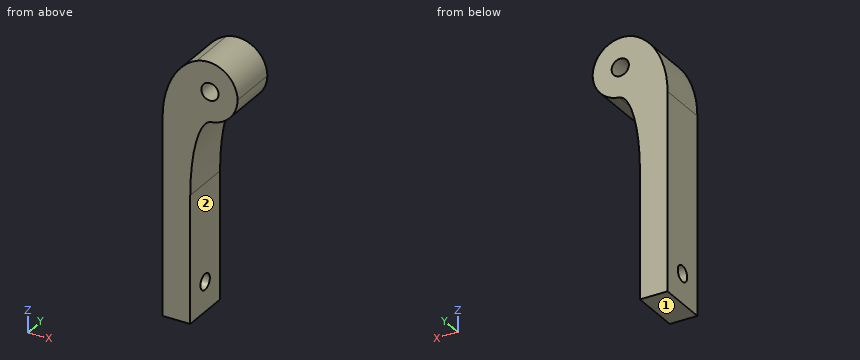
from build123d import *

# Parameters (mm, degrees)
SKETCH1_W               = 7
SKETCH1_H               = 52
BOSS_EXTRUDE1_DEPTH     = 12.7
SKETCH2_R               = 2
CUT_EXTRUDE1_DEPTH      = 10
SKETCH3_W               = 24
SKETCH3_H               = 15
BOSS_EXTRUDE2_DEPTH     = 12.7
CUT_EXTRUDE2_DEPTH      = 48.566164445
CUT_EXTRUDE2_DEPTH_BACK = 48.566164445
SKETCH4_R               = 2.1844
FILLET1_SIZE            = 17
FILLET1_SIZE_2          = 12
CUT_EXTRUDE3_DEPTH      = 48.566164601
CUT_EXTRUDE3_DEPTH_BACK = 48.566164601
SKETCH5_W               = 5
SKETCH5_H               = 15
FILLET2_R               = 7.5
FILLET3_DEPTH           = 12.7


with BuildPart() as part:
    # Sketch1 → Boss-Extrude1 (new body)
    with BuildSketch(Plane(origin=(0, 0, 0), x_dir=(1, 0, 0), z_dir=(0, 1, 0))):
        Rectangle(SKETCH1_W, SKETCH1_H)
    extrude(amount=BOSS_EXTRUDE1_DEPTH)

    # Sketch2 → Cut-Extrude1 (cut)
    with BuildSketch(Plane.ZY.offset(3.5)):
        with Locations((-18.5, 6.35)):
            Circle(SKETCH2_R)
    extrude(amount=-CUT_EXTRUDE1_DEPTH, mode=Mode.SUBTRACT)

    # Sketch3 → Boss-Extrude2 (add)
    with BuildSketch(Plane.XZ):
        with Locations((8.5, 33.5)):
            Rectangle(SKETCH3_W, SKETCH3_H)
    extrude(amount=-BOSS_EXTRUDE2_DEPTH)

    # Sketch4 → Cut-Extrude2 (cut, two sides: drawn at the far end of the back side and taken through both)
    with BuildSketch(Plane(origin=(0, 12.7, 0), x_dir=(1, 0, 0), z_dir=(0, 1, 0)).offset(-CUT_EXTRUDE2_DEPTH_BACK)):
        with Locations(Location((8.5, -33.5, 0), (0, 0, 270))):
            Circle(SKETCH4_R)
    extrude(amount=CUT_EXTRUDE2_DEPTH + CUT_EXTRUDE2_DEPTH_BACK, mode=Mode.SUBTRACT)

    # Fillet1
    # a fillet whose section is not a circle: 17, 12 mm, written as the material it takes off along each edge
    with BuildSketch(Plane(origin=(-3.5, -42.5, 41), x_dir=(0, 0, -1), z_dir=(0, 1, 0))) as fillet1_piece_1:
        with BuildLine():
            Bezier((FILLET1_SIZE, 0), (0, 0), (0, -FILLET1_SIZE_2), weights=[1, 0.707106781, 1])
            Line((0, -FILLET1_SIZE_2), (0, 0))
            Line((0, 0), (FILLET1_SIZE, 0))
        make_face()
    extrude(amount=97.7, mode=Mode.SUBTRACT)

    # Sketch5 → Cut-Extrude3 (cut, two sides: drawn at the far end of the back side and taken through both)
    with BuildSketch(Plane(origin=(0, 12.7, 0), x_dir=(1, 0, 0), z_dir=(0, 1, 0)).offset(-CUT_EXTRUDE3_DEPTH_BACK)):
        with Locations((18, -33.5)):
            Rectangle(SKETCH5_W, SKETCH5_H)
    extrude(amount=CUT_EXTRUDE3_DEPTH + CUT_EXTRUDE3_DEPTH_BACK, mode=Mode.SUBTRACT)

    # Fillet2
    # the kernel refuses this fillet: 7.5 mm, written as the material it takes off along each edge
    with BuildSketch(Plane(origin=(15.5, -18.75, 26), x_dir=(-1, 0, 0), z_dir=(0, 1, 0))) as fillet2_piece_1:
        with BuildLine():
            CenterArc((FILLET2_R, FILLET2_R), FILLET2_R, 180, 90)
            Line((0, FILLET2_R), (0, 0))
            Line((0, 0), (FILLET2_R, 0))
        make_face()
    extrude(amount=50.2, mode=Mode.SUBTRACT)
    with BuildSketch(Plane(origin=(15.5, -26.005596716, 41), x_dir=(-0.9978099648287924, 0, -0.06614585465744831), z_dir=(0, 1, 0))) as fillet2_piece_2:
        with BuildLine():
            CenterArc((7.98716223, -7.10052151), FILLET2_R, 71.215463445, 112.577183941)
            Line((0.503587494, -7.59661542), (-0.24476998, -7.646224811))
            Line((-0.24476998, -7.646224811), (-0.748357474, -0.049609391))
            Line((-0.748357474, -0.049609391), (-0.049609391, 0.748357474))
            ThreePointArc((-0.049609391, 0.748357474), (6.935060363, 1.211378456), (10.643746332, 0.710052151))
            Line((10.643746332, 0.710052151), (10.402238686, 0))
        make_face()
    extrude(amount=64.711193432, mode=Mode.SUBTRACT)

    # Fillet3: read off the stored shape, not the designer's step
    # Fillet3 outline → Fillet3 (add)
    with BuildSketch(Plane(origin=(0, 0, 0), x_dir=(1, 0, 0), z_dir=(0, 1, 0))):
        with BuildLine():
            add(Edge.make_bspline(
                [(3.5, -6.164126134), (3.5, -25.461113038), (8.818181818, -26.044761673)],
                knots=[0, 0, 0, 1, 1, 1], degree=2, weights=[1, 0.744678088, 1]))
            Line((3.5, -6.164126134), (3.5, -26))
            Line((3.5, -26), (8, -26))
            ThreePointArc((8, -26), (8.409702665, -26.011198779), (8.818181818, -26.044761673))
        make_face()
    extrude(amount=FILLET3_DEPTH)


solid = part.part
Geometry: final body of the model. Coordinates: model frame, mm. Face numbers are marked on the shaded views. A direction names the side the tool comes from. Round coordinates to 2 decimals unless told otherwise and drop trailing zeros. Loops run counter-clockwise (first coordinate to the right, second up) from the corner with the lowest first, then second, coordinate; pieces in that order, holes last.
Q1. Access query for the marked faces 1 and 2. Directions: +Z, -Z, +X, -X, +Y, -Y. A direction counts if a zero-diameter tool reaches every point of the face in a straight line with its end or side. Return the directions, or none.
Q2. Section A-A on z = -18.5. Return loops of the section in (x, y).
Q3. Section C-C on x = 9.75. Return loops of the section in (y, z), plus the area to 3 significant figures.
Q4. Material intervals for L1, parallel to Y at x = -0.75, z = -18.5; L2, parallel to Z at x = 8.5, y = 5.25; L3, parallel to Z at x = 8.25, y = 7.25, sorted ascending.
Q5. Section B-B on y = 6.35. State how many separate pieces and enclosed holes the cut face has, plus the area to 3 significant figures.
Q6. Pin query (flat end, axial travel): P1, Ø2, axis at y = 11, z = -4, coming from the +X side; P2, Ø3.5, axis at y = 6.35, z = -18.5, coming from the +X side. Return the tip coordinate at first contact, or that it passes through.
Evaluation:
1. face 1: -Z, +X, -X, +Y, -Y
1. face 2: -Z, +X, +Y, -Y
2. outline: (-3.5, 0) - (3.5, 0) - (3.5, 4.35) - (-3.5, 4.35) - close; (-3.5, 8.35) - (3.5, 8.35) - (3.5, 12.7) - (-3.5, 12.7) - close
3. outline: (0, 26.21) - (12.7, 26.21) - (12.7, 31.71) - (0, 31.71) - close; (0, 35.29) - (12.7, 35.29) - (12.7, 40.68) - (0, 40.68) - close
3. area: 138 mm2
4. L1: y = 0 to 4.35, 8.35 to 12.7
4. L2: z = 25.98 to 31.32, 35.68 to 40.87
4. L3: z = 25.88 to 31.33, 35.67 to 40.88
5. separate pieces: 2
5. enclosed holes: 1
5. area: 560 mm2
6. P1: stops at x = 3.5
6. P2: passes through
